Can you work these out from the model? Positions are in its coordinate system, mm. A direction names the side the tool comes from. Coordinates: 2 decimals unless noted, no trailing zeros. Order: outer loops, then holes, each group sorted by start corner. A loop starts at its lowest first (then second) coordinate and runs counter-clockwise, first axis right, second up. Notation, with made-up numbers: (5, 31.5) - (26, 31.5) arc R22 ccw to (26, 41.5) - close; hole circle Ø1 at (67, 23). An arc over 180 degrees is marked (long way). Return JSON: item names as keys, results as strings. Group by question number.
1) If I drill on line 1 along Z through (x, y) = (81, 26.75); line 2 along Z through (x, y) = (26, 29); line 3 along Y through (x, z) = (107, 52), over which ranges is the centre line in solid material (lowest first)?
2) Imagine slicing it at D-D (z = 49). Write out the boundary of the cut face in (x, y), and give its area (3 significant figures).
3) If we mould it in two halves opening along X, with no side actions, what happens to faces 4 (the face through (93, 14, 54)), 5 (the face through (111.619, 12.085, 54.302)), 6 (the face through (134.69, 19.68, 15.93))? For each: pulls with the +X half, pulls with the -X half, needs draft (parallel to the pull), parting line crosses it, or undercut.
4) Imagine slicing it at C-C (y = 23.5). Write out the boundary of the cut face in (x, z).
5) Which directions (+Z, -Z, +X, -X, +Y, -Y) give clear straight access to the entire face, cutting with the end or side of a thin tool? Please do faces 1 (the face through (121, 20, 7)), 2 (the face through (135.7, 20.3, 46.6)), 3 (the face through (10.175, 28.697, 43.036)).
6) Imagine slicing it at A-A (z = 33). Write out the boundary of the cut face in (x, y), and give its area (3 significant figures).
7) Imagine slicing it at B-B (x = 41.5). Write out the boundary of the cut face in (y, z).
8) For pin 1 Ø13 at (x, y) = (107, 14) entering from -Z; pin 2 Ø10.5 at (x, z) = (136.5, 50) entering from -Y; pin 3 Ø6.5 at (x, z) = (81, 20) entering from +Y; pin 4 Ø3.5 at (x, z) = (41.5, 44.5) entering from -Y, each with a flat end and sliding along its axis, tell me the tip position at first contact or that it passes through.
```python
from build123d import *

# Parameters (mm, degrees)
PAD_DEPTH       = 58
SKETCH001_R     = 4
POCKET_DEPTH    = 25
SKETCH002_W     = 28
SKETCH002_H     = 25
POCKET001_DEPTH = 50.5
POCKET002_DEPTH = 27
SKETCH004_R     = 5
SKETCH004_R_2   = 1.5
POCKET003_DEPTH = 58.001
SKETCH005_R     = 12
SKETCH005_R_2   = 1.5
SKETCH005_R_3   = 2
POCKET004_DEPTH = 7.501
CHAMFER_SIZE    = 2
CHAMFER001_SIZE = 3
CHAMFER002_SIZE = 3


with BuildPart() as part:
    # Sketch → Pad (new body)
    with BuildSketch(Plane.XY):
        Polygon((0, 25), (0, 32.5), (148, 32.5), (148, 14.5), (121, 14.5), (121, 0), (93, 0), (93, 25), align=None)
    extrude(amount=PAD_DEPTH)

    # Sketch001 (on Face3 of Pad) → Pocket (cut)
    with BuildSketch(Plane.YZ.offset(148)):
        with Locations((23.5, 49)):
            Circle(SKETCH001_R)
        with Locations((23.5, 9)):
            Circle(SKETCH001_R)
    extrude(amount=-POCKET_DEPTH, mode=Mode.SUBTRACT)

    # Sketch002 (on Face4 of Pocket) → Pocket001 (cut)
    with BuildSketch(Plane(origin=(0, 0, 0), x_dir=(1, 0, 0), z_dir=(0, 0, -1))):
        with Locations((107, -12.5)):
            Rectangle(SKETCH002_W, SKETCH002_H)
    extrude(amount=-POCKET001_DEPTH, mode=Mode.SUBTRACT)

    # Sketch003 (on Face8 of Pocket001) → Pocket002 (cut)
    with BuildSketch(Plane.YZ.offset(148)):
        Polygon((14.5, 45.062178), (14.5, 12.937822), (25, 19), (25, 39), align=None)
    extrude(amount=-POCKET002_DEPTH, mode=Mode.SUBTRACT)

    # Sketch004 (on Face4 of Pocket002) → Pocket003 (cut, through all)
    with BuildSketch(Plane.XY.offset(58)):
        with Locations((107, 14)):
            Circle(SKETCH004_R)
        with Locations((101.343146, 19.656854)):
            Circle(SKETCH004_R_2)
        with Locations((112.656854, 19.656854)):
            Circle(SKETCH004_R_2)
        with Locations((112.656854, 8.343146)):
            Circle(SKETCH004_R_2)
        with Locations((101.343146, 8.343146)):
            Circle(SKETCH004_R_2)
    extrude(amount=-POCKET003_DEPTH, mode=Mode.SUBTRACT)

    # Sketch005 (on Face2 of Pocket003) → Pocket004 (cut, through all)
    with BuildSketch(Plane.XZ.offset(-25)):
        with Locations((26, 29)):
            Circle(SKETCH005_R)
        with Locations((10.5, 44.5)):
            Circle(SKETCH005_R_2)
        with Locations((41.5, 44.5)):
            Circle(SKETCH005_R_2)
        with Locations((10.5, 13.5)):
            Circle(SKETCH005_R_2)
        with Locations((41.5, 13.5)):
            Circle(SKETCH005_R_2)
        with Locations((57, 38)):
            Circle(SKETCH005_R_3)
        with Locations((81, 38)):
            Circle(SKETCH005_R_3)
        with Locations((81, 20)):
            Circle(SKETCH005_R_3)
        with Locations((57, 20)):
            Circle(SKETCH005_R_3)
    extrude(amount=-POCKET004_DEPTH, mode=Mode.SUBTRACT)

    # Chamfer
    chamfer_edges = [part.edges().sort_by_distance(p)[0] for p in [
        (148, 23.5, 58),
        (148, 23.5, 0),
    ]]
    chamfer(chamfer_edges, length=CHAMFER_SIZE)

    # Chamfer001
    chamfer001_edges = [part.edges().sort_by_distance(p)[0] for p in [
        (121, 0, 54.25),
        (93, 0, 54.25),
    ]]
    chamfer(chamfer001_edges, length=CHAMFER001_SIZE)

    # Chamfer002
    chamfer002_edges = [part.edges().sort_by_distance(p)[0] for p in [
        (0, 28.75, 58),
        (0, 28.75, 0),
    ]]
    chamfer(chamfer002_edges, length=CHAMFER002_SIZE)


solid = part.part
```
Calculated:
{
 "1": {"line 1": "0 to 18, 22 to 36, 40 to 58", "line 2": "0 to 17, 41 to 58", "line 3": "0 to 9, 19 to 32.5"},
 "2": {"outline": "(0, 25) - (121, 25) - (121, 14.5) - (148, 14.5) - (148, 19.5) - (123, 19.5) - (123, 27.5) - (148, 27.5) - (148, 32.5) - (0, 32.5) - close", "area": "1,190 mm2"},
 "3": {"face 4": "pulls with the -X half", "face 5": "undercut", "face 6": "needs draft"},
 "4": {"outline": "(93, 50.5) - (121, 50.5) - (121, 39.87) - (148, 39.87) - (148, 45) - (123, 45) - (123, 53) - (148, 53) - (148, 56) - (146, 58) - (93, 58) - close; (121, 0) - (146, 0) - (148, 2) - (148, 5) - (123, 5) - (123, 13) - (148, 13) - (148, 18.13) - (121, 18.13) - close"},
 "5": {"face 1": "-Z, -X, -Y", "face 2": "+X", "face 3": "+Y, -Y"},
 "6": {"outline": "(0, 25) - (14.69, 25) - (14.69, 32.5) - (0, 32.5) - close; (37.31, 25) - (148, 25) - (148, 32.5) - (37.31, 32.5) - close", "area": "940 mm2"},
 "7": {"outline": "(25, 0) - (32.5, 0) - (32.5, 12) - (25, 12) - close; (25, 15) - (32.5, 15) - (32.5, 43) - (25, 43) - close; (25, 46) - (32.5, 46) - (32.5, 58) - (25, 58) - close"},
 "8": {"pin 1": "z = 50.5", "pin 2": "y = 14.5", "pin 3": "y = 32.5", "pin 4": "y = 25"}
}
